Input: dimensioned drawing with shaded views. Units: mm. Origin: part minimum x, y, z. A direction names the side the tool comes from. Round coordinates to 2 decimals unless told otherwise and drop trailing zeros. Write each loop counter-clockwise with the first axis right and the second up, starting at its lowest first coordinate (ties: lowest second). Pieces come first, ordered by that corner, then holes. Notation, with made-up numbers: (-23.75, -26) -> (-9.75, -26) arc R15 cw to (-9.75, -11) -> close; hole circle Ø10 at (-37, 23.25). An arc over 180 degrees is marked (long way). Return JSON: item names as keys, results as strings. Group by question number.
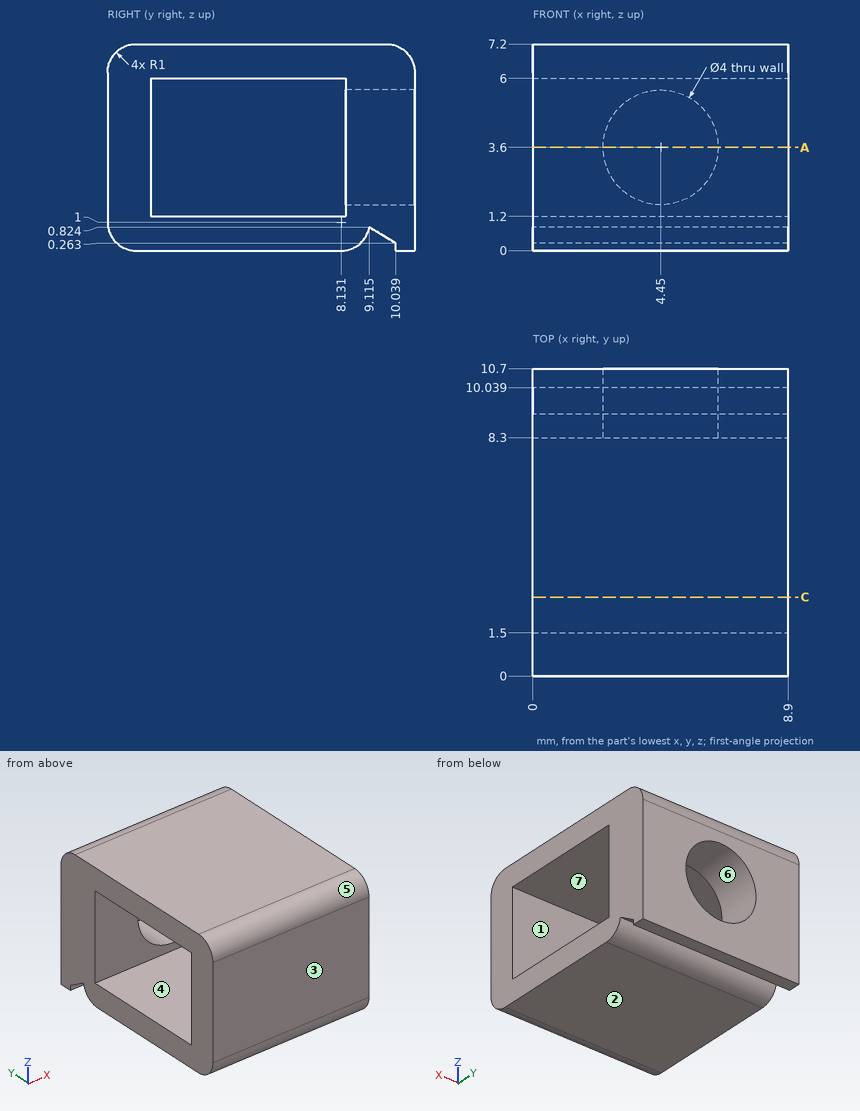
Item 1: Pull-direction query (Y, two-part tool) for the marked faces 1, 2, 3 and 4; classes: +Y half, -Y half, draft (parallel to the pull), parting line (faces both ways), or undercut.
Item 2: Set-up query: the marked faces 5, 6 and 7. Return all of +Z, -Z, +X, -X, +Y, -Y with unobstructed straight access to the full face (end or side cutting, diameter ignored); none if empty.
Item 3: Material intervals for probe 1 along Z at (x, y) = (6.5, 3); probe 2 along X at (y, z) = (9.3, 3.6); probe 3 along Y at (x, z) = (1.25, 4.5), sorted ascending.
Item 4: Cut plane A-A on z = 3.6. Output: boundary loops of the cut face in (x, y).
Item 5: Cut plane C-C on y = 2.75. Output: boundary loops of the cut face in (x, z).
Item 6: First-contact query: pin 1 Ø3 at (y, z) = (4.5, 2) entering from -X. Flat tip, straight axial feed; report the tip coordinate or a pass-through.
Here are the results:
{
 "1": {"face 1": "undercut", "face 2": "draft", "face 3": "-Y half", "face 4": "undercut"},
 "2": {"face 5": "+Z, +X, -X, -Y", "face 6": "+Y", "face 7": "+X, -X"},
 "3": {"probe 1": "z = 0 to 1.2, 6 to 7.2", "probe 2": "x = 0 to 2.45, 6.45 to 8.9", "probe 3": "y = 0 to 1.5, 8.3 to 10.7"},
 "4": {"outline": "(0, 0) -> (8.9, 0) -> (8.9, 1.5) -> (0, 1.5) -> close; (0, 8.3) -> (2.45, 8.3) -> (2.45, 10.7) -> (0, 10.7) -> close; (6.45, 8.3) -> (8.9, 8.3) -> (8.9, 10.7) -> (6.45, 10.7) -> close"},
 "5": {"outline": "(0, 0) -> (8.9, 0) -> (8.9, 1.2) -> (0, 1.2) -> close; (0, 6) -> (8.9, 6) -> (8.9, 7.2) -> (0, 7.2) -> close"},
 "6": {"pin 1": "stops at x = 0"}
}
